```python
from build123d import *

# Parameters (mm, degrees)
SKETCH1_W           = 100
SKETCH1_H           = 20
BOSS_EXTRUDE1_DEPTH = 100
SKETCH2_W           = 90
SKETCH2_H           = 15
BOSS_EXTRUDE2_DEPTH = 45
CUT_EXTRUDE1_DEPTH  = 86


with BuildPart() as part:
    # Sketch1 → Boss-Extrude1 (new body)
    with BuildSketch(Plane.XY):
        with Locations((25, -30)):
            Rectangle(SKETCH1_W, SKETCH1_H)
        with BuildLine():
            ThreePointArc((-60, 17.087121525), (-70.916500663, 26.306936062), (-75, 40))
            Line((-75, 40), (-75, -40))
            Line((-75, -40), (-25, -40))
            Line((-25, -40), (-25, -20))
            Line((-25, -20), (-25, 40))
            ThreePointArc((-25, 40), (-29.083499337, 26.306936062), (-40, 17.087121525))
            Line((-40, 17.087121525), (-40, -15))
            ThreePointArc((-40, -15), (-50, -25), (-60, -15))
            Line((-60, -15), (-60, 17.087121525))
        make_face()
        with BuildLine():
            ThreePointArc((-40, 17.087121525), (-29.083499337, 26.306936062), (-25, 40))
            Line((-25, 40), (-40, 40))
            Line((-40, 40), (-40, 17.087121525))
        make_face()
        with BuildLine():
            ThreePointArc((-25, 40), (-50, 65), (-75, 40))
            Line((-75, 40), (-60, 40))
            ThreePointArc((-60, 40), (-50, 50), (-40, 40))
            Line((-40, 40), (-25, 40))
        make_face()
        with BuildLine():
            Line((-60, 40), (-75, 40))
            ThreePointArc((-75, 40), (-70.916500663, 26.306936062), (-60, 17.087121525))
            Line((-60, 17.087121525), (-60, 40))
        make_face()
    extrude(amount=BOSS_EXTRUDE1_DEPTH)

    # Sketch2 → Boss-Extrude2 (add)
    with BuildSketch(Plane(origin=(0, -20, 0), x_dir=(1, 0, 0), z_dir=(0, 1, 0))):
        with Locations((20, -77.5)):
            Rectangle(SKETCH2_W, SKETCH2_H)
        with Locations((20, -22.5)):
            Rectangle(SKETCH2_W, SKETCH2_H)
    extrude(amount=BOSS_EXTRUDE2_DEPTH)

    # Sketch3 → Cut-Extrude1 (cut, through all)
    with BuildSketch(Plane.XY.offset(85)):
        Polygon((-25, 25), (65, -20), (65, 25), align=None)
    extrude(amount=-CUT_EXTRUDE1_DEPTH, mode=Mode.SUBTRACT)


solid = part.part
```
Input: part model. Units: mm. Frame: model coordinates. A direction names the side the tool comes from. Round coordinates to 2 decimals unless told otherwise and drop trailing zeros. Loops run counter-clockwise (first coordinate to the right, second up) from the corner with the lowest first, then second, coordinate; pieces in that order, holes last. Notation, with made-up numbers: M -26.5,51.25 L 18.5,51.25 A13 ccw 18.5,65.25 Z; hole C 13,55.25 d9. An arc over 180 degrees is marked long. Answer in a Markdown table with one row per item. Add a question column.
1. Section C-C (z = 88.5). Output: boundary loops of the cut face in (x, y), and give its area (3 significant figures).
2. Contact query for flat-ended pins moving along their axis: pin 1 (12 mm diameter, centred on y = -12, z = 44.5, fed in from +X); pin 2 (22.5 mm diameter, centred on x = 16.5, y = -0.5, fed in from +Z); pin 3 (4 mm diameter, centred on x = -11, z = 14, fed in from +Y). Output: stop coordinate, or through.
3. Ray query, probe 1 along Z at (x, y) = (-20, 4.5); probe 2 along X at (y, z) = (9.5, 48.5); probe 3 along Y at (x, z) = (10, 69). Return the intervals inside material, ascending.
4. Section A-A (y = 1.5). Output: boundary loops of the cut face in (x, z).
5. Set-up query: faces 1 (the face through (9, -3, 30)), 2 (the face through (9, -3, 85)), 3 (the face through (9, -3, 15)). Return all of +Z, -Z, +X, -X, +Y, -Y with unobstructed straight access to the full face (end or side cutting, diameter ignored); none if empty.
6. Section D-D (x = -2). Output: boundary loops of the cut face in (y, z).
7. Mould query, pull axis X, two halves, no side actions, for faces 4 (the face through (-40, 13, 49)), 5 (the face through (-50, -25, 49)), 6 (the face through (-25, 16, 49)), 7 (the face through (24, -20, 49)). Classes: released by +X, released by -X, zero draft, split by the parting line, or undercut.
8. Section B-B (x = -50). Output: boundary loops of the cut face in (y, z).
Values follow:
| question | item | result |
|---|---|---|
| 1 | outline | M -75,-40 L 75,-40 L 75,-20 L -25,-20 L -25,40 A25 ccw -75,40 Z; hole M -60,-15 A10 ccw -40,-15 L -40,40 A10 ccw -60,40 Z |
| 1 | area | 5,570 mm^2 |
| 2 | pin 1 | x = -25 |
| 2 | pin 2 | z = 85 |
| 2 | pin 3 | y = 18.87 |
| 3 | probe 1 | 15 to 30, 70 to 85 |
| 3 | probe 2 | -75 to -60, -40 to -25 |
| 3 | probe 3 | -40 to -20 |
| 4 | outline | M -75,0 L -60,0 L -60,100 L -75,100 Z; M -40,0 L -25,0 L -25,15 L 22,15 L 22,30 L -25,30 L -25,70 L 22,70 L 22,85 L -25,85 L -25,100 L -40,100 Z |
| 5 | face 1 | +X, +Y |
| 5 | face 2 | +Z, +X, +Y |
| 5 | face 3 | -Z, +X, +Y |
| 6 | outline | M -40,0 L -20,0 L -20,15 L 13.5,15 L 13.5,30 L -20,30 L -20,70 L 13.5,70 L 13.5,85 L -20,85 L -20,100 L -40,100 Z |
| 7 | face 4 | undercut |
| 7 | face 5 | undercut |
| 7 | face 6 | released by +X |
| 7 | face 7 | zero draft |
| 8 | outline | M -40,0 L -25,0 L -25,100 L -40,100 Z; M 50,0 L 65,0 L 65,100 L 50,100 Z |
